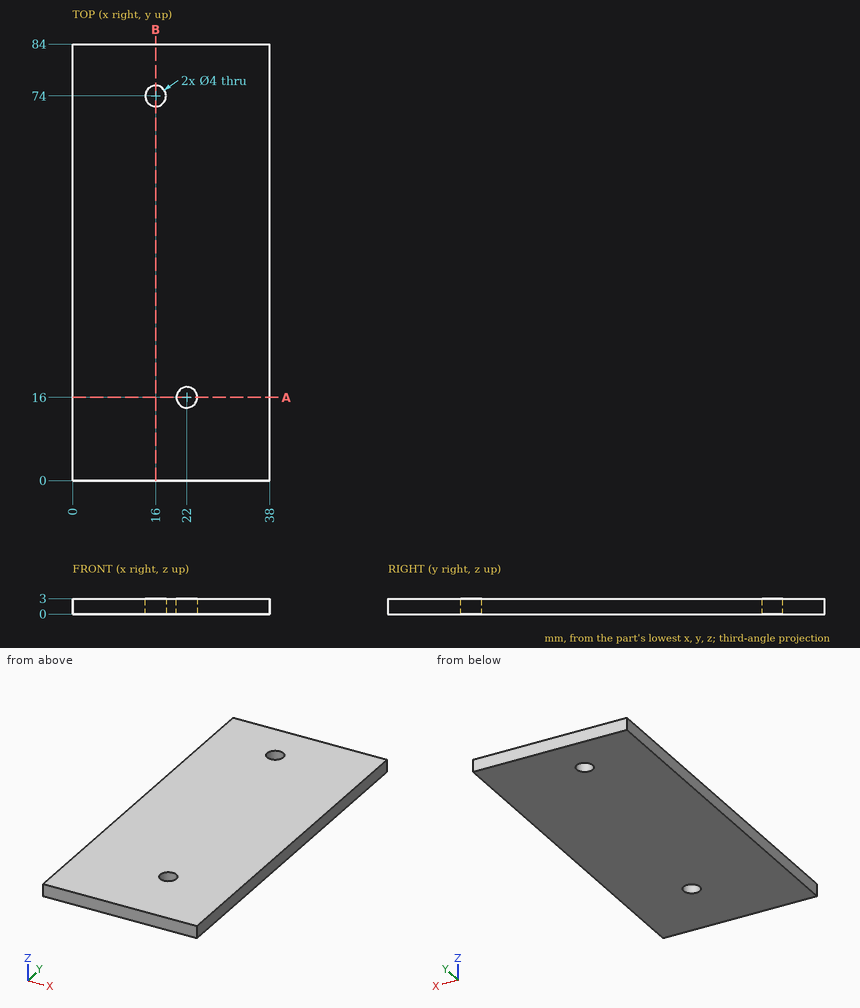
Part print with two shaded views. Sizes in mm from the minimum x, y, z corner. Coordinates: 2 decimals unless noted, no trailing zeros. Write each loop counter-clockwise with the first axis right and the second up, starting at its lowest first coordinate (ties: lowest second). Pieces come first, ordered by that corner, then holes. Notation, with made-up numbers: M 30,45.25 L 77,45.25 A27 cw 77,83.25 Z; hole C 11.5,39 d1. An arc over 180 degrees is marked long. Return JSON: item names as keys, results as strings.
Item 1: Probe line 1 (Y direction, x = 16, z = 0.7); line 2 (Y direction, x = 22, z = 2.15). List the from-to ranges inside material, lowest first. Write a range as from..to.
Findings below:
{"line 1": "y = 0..72, 76..84", "line 2": "y = 0..14, 18..84"}
Item 2: Drop a flat-ended pin along its axis: pin 1 Ø3.5 at (x, y) = (22, 16) entering from -Z. Give the stop position or say it passes through.
Findings below:
{"pin 1": "passes through"}
Item 3: Slice it at B-B, the plane x = 16. Write the cut outline in (y, z).
Findings below:
{"outline": "M 0,0 L 72,0 L 72,3 L 0,3 Z; M 76,0 L 84,0 L 84,3 L 76,3 Z"}
Item 4: Slice it at A-A, the plane y = 16. Write the cut outline in (x, z), and give its area (3 significant figures).
Findings below:
{"outline": "M 0,0 L 20,0 L 20,3 L 0,3 Z; M 24,0 L 38,0 L 38,3 L 24,3 Z", "area": "102 mm2"}
